Check sheet for the drawn part. Datum: minimum x, y, z corner. Units: mm. A direction names the side the tool comes from. Round coordinates to 2 decimals unless told otherwise and drop trailing zeros. Loops run counter-clockwise (first coordinate to the right, second up) from the corner with the lowest first, then second, coordinate; pieces in that order, holes last. Notation, with made-up numbers: (-4, -5) - (42, -5) arc R9 ccw to (42, 2) - close; hole circle Ø2 at (-18, -18). An arc over 180 degrees is marked (long way). Use CSV: the item, a comma, the result in double quotes.
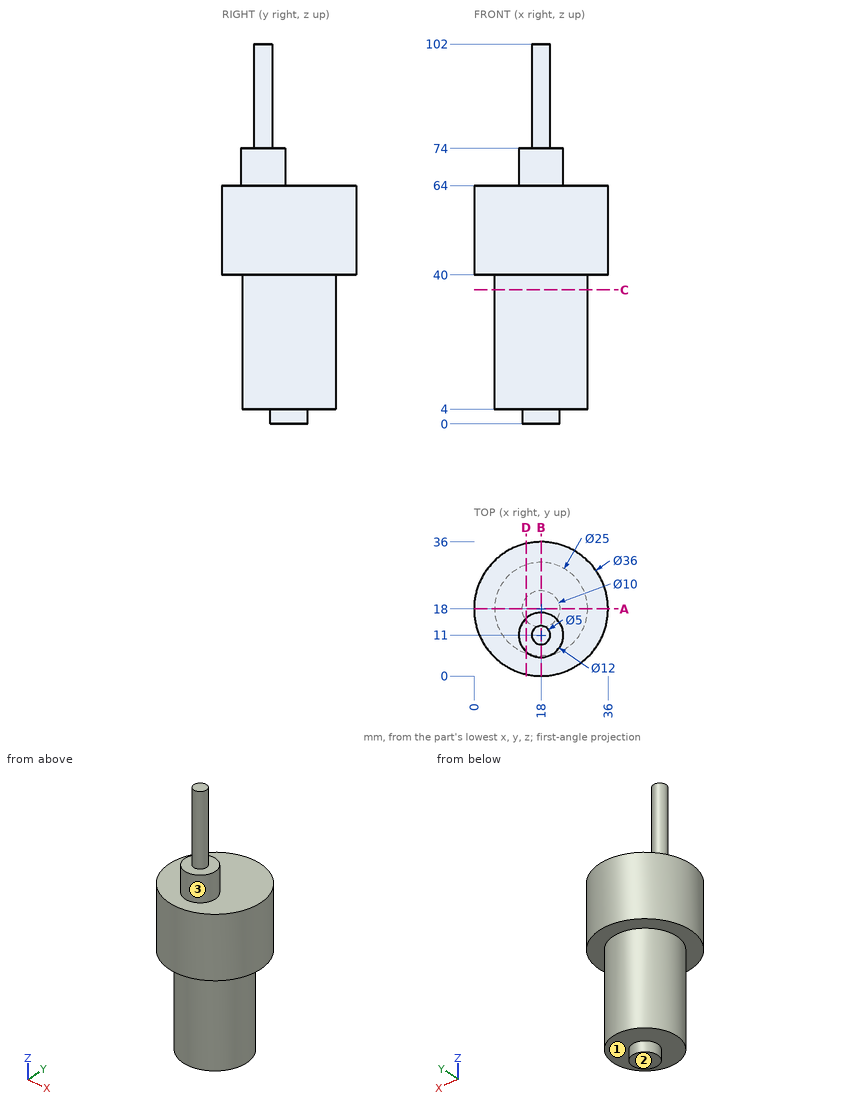
1) Gauge pin test, flat ends, axial feed: pin 1 Ø6 at (x, y) = (11.5, 28.5) entering from +Z; pin 2 Ø5 at (x, z) = (11.5, 75.5) entering from -Y; pin 3 Ø2 at (x, z) = (21.5, 42.5) entering from -Y. Record the tip position at first contact, or that the pin passes through.
Returned:
pin 1,"stops at z = 64"
pin 2,"stops at y = 7.03"
pin 3,"stops at y = 0.17"
2) Thickness scan on probe 1 along Y at (x, z) = (18.5, 16.5); probe 2 along Z at (x, y) = (26, 20); probe 3 along Z at (x, y) = (16, 11). Record the ranges inside material, lowest first. Write a range as [from, to].
Returned:
probe 1,"y = [5.51, 30.49]"
probe 2,"z = [4, 64]"
probe 3,"z = [4, 102]"
3) Cross-section at C-C, the plane z = 36. Record the cut outline in (x, y), then the cut area to 3 significant figures.
Returned:
outline,"circle Ø25 at (18, 18)"
area,"491 mm²"
4) Cross-section at D-D, the plane x = 14. Record the cut outline in (y, z).
Returned:
outline,"(0.45, 40) - (6.16, 40) - (6.16, 4) - (15, 4) - (15, 0) - (21, 0) - (21, 4) - (29.84, 4) - (29.84, 40) - (35.55, 40) - (35.55, 64) - (15.47, 64) - (15.47, 74) - (6.53, 74) - (6.53, 64) - (0.45, 64) - close"
5) Cross-section at B-B, the plane x = 18. Record the cut outline in (y, z), then the cut area to 3 significant figures.
Returned:
outline,"(0, 40) - (5.5, 40) - (5.5, 4) - (13, 4) - (13, 0) - (23, 0) - (23, 4) - (30.5, 4) - (30.5, 40) - (36, 40) - (36, 64) - (17, 64) - (17, 74) - (13.5, 74) - (13.5, 102) - (8.5, 102) - (8.5, 74) - (5, 74) - (5, 64) - (0, 64) - close"
area,"2,060 mm²"
6) Access from +Z, -Z, +X, -X, +Y, -Y to the whole of each face (thin tool, end or side, straight path). Record for the marked faces 1, 2 and 3.
Returned:
face 1,"-Z"
face 2,"-Z, +X, -X, +Y, -Y"
face 3,"+Z"
7) Cross-section at A-A, the plane y = 18. Record the cut outline in (x, z), then the cut area to 3 significant figures.
Returned:
outline,"(0, 40) - (5.5, 40) - (5.5, 4) - (13, 4) - (13, 0) - (23, 0) - (23, 4) - (30.5, 4) - (30.5, 40) - (36, 40) - (36, 64) - (0, 64) - close"
area,"1,800 mm²"
